from build123d import *

# Parameters (mm, degrees)
SKETCH063_W      = 2
SKETCH063_H      = 2
EXTRUDE068_DEPTH = 3.8
SKETCH062_W      = 2
SKETCH062_H      = 6.2
EXTRUDE067_DEPTH = 6.4
SKETCH061_W      = 2
SKETCH061_H      = 10.2
EXTRUDE066_DEPTH = 8.4


with BuildPart() as obj1:
    # Sketch063 → Extrude068 (new body, symmetric)
    with BuildSketch(Plane.XZ):
        with Locations((-2, 4.1)):
            Rectangle(SKETCH063_W, SKETCH063_H)
        with Locations((-2, -4.1)):
            Rectangle(SKETCH063_W, SKETCH063_H)
    extrude(amount=EXTRUDE068_DEPTH, both=True)


with BuildPart() as obj2:
    # Sketch062 → Extrude067 (new body, symmetric)
    with BuildSketch(Plane.XZ):
        Rectangle(SKETCH062_W, SKETCH062_H)
    extrude(amount=EXTRUDE067_DEPTH, both=True)


with BuildPart() as obj3:
    # Sketch061 → Extrude066 (new body, symmetric)
    with BuildSketch(Plane.XZ):
        Rectangle(SKETCH061_W, SKETCH061_H)
    extrude(amount=EXTRUDE066_DEPTH, both=True)

    # Cut036: cut obj2
    add(obj2.part, mode=Mode.SUBTRACT)

    # Fusion002: union obj1
    add(obj1.part)


solid = obj3.part
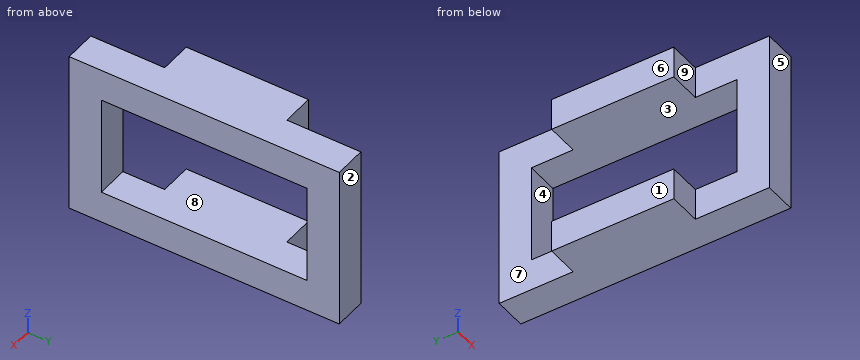
Read the model definition and answer for the solid it produces. Units are mm, in the model's axes. Face numbers are marked on the shaded views. A direction names the side the tool comes from. Round coordinates to 2 decimals unless told otherwise and drop trailing zeros. Loops run counter-clockwise (first coordinate to the right, second up) from the corner with the lowest first, then second, coordinate; pieces in that order, holes last.
Q1. Section B-B on x = 0.5 is taken. Write down the section's boundary in (y, z).
Q2. Each of these flat-tipped pins is pushed along its axis until it touches: pin 1 (2 mm diameter, centred on x = -1.5, z = -4, fed in from +Y); pin 2 (0.6 mm diameter, centred on x = -2.5, z = 4, fed in from +Y); pin 3 (1.4 mm diameter, centred on y = -6.5, z = 0, fed in from -X); pin 4 (2 mm diameter, centred on x = -2.5, z = -4.5, fed in from -Y). Where does it stop, or does it pass through?
Q3. Which of the six approach directions +Z, -Z, +X, -X, +Y, -Y give full straight-line access (tool end or side, diameter ignored) to the marked faces 5, 6, 7, 8 and 9?
Q4. Section D-D on z = -3.75 is taken. Write down the section's boundary in (x, y), and give its area (3 significant figures).
Q5. Section A-A on y = -5.5 is taken. Write down the section's boundary in (x, z).
Q6. Section C-C on z = -2.5 is taken. Write down the section's boundary in (x, y).
Q7. Consider probe 1 along Z at (x, y) = (-1.5, -2); probe 2 along Y at (x, z) = (-0.9, -2.75); probe 3 along X at (y, z) = (-6.75, 4). Determine where each line is inside the solid, lowest interval first.
Q8. Determine the mould class of the marked faces 1, 2, 3 and 4 for opening direction Y: released by +Y, released by -Y, zero draft, split by the parting line, or undercut.
Output:
1. outline: (-8.4, -5.1) - (8.4, -5.1) - (8.4, 5.1) - (-8.4, 5.1) - close; hole (-6.4, -3.1) - (6.4, -3.1) - (6.4, 3.1) - (-6.4, 3.1) - close
2. pin 1: stops at y = 8.4
2. pin 2: stops at y = 3.8
2. pin 3: stops at x = -1
2. pin 4: stops at y = -3.8
3. face 5: +Z, -Z, +X, -X, -Y
3. face 6: +Z, -Z, -X, +Y, -Y
3. face 7: +Z, -Z, -X, +Y
3. face 8: +X, -X
3. face 9: +Z, -Z, -X, -Y
4. outline: (-3, -3.8) - (-1, -3.8) - (-1, -8.4) - (1, -8.4) - (1, 8.4) - (-1, 8.4) - (-1, 3.8) - (-3, 3.8) - close
4. area: 48.8 mm2
5. outline: (-1, -5.1) - (1, -5.1) - (1, -3.1) - (-1, -3.1) - close; (-1, 3.1) - (1, 3.1) - (1, 5.1) - (-1, 5.1) - close
6. outline: (-1, -8.4) - (1, -8.4) - (1, -6.4) - (-1, -6.4) - close; (-1, 6.4) - (1, 6.4) - (1, 8.4) - (-1, 8.4) - close
7. probe 1: z = -5.1 to -3.1, 3.1 to 5.1
7. probe 2: y = -8.4 to -6.4, 6.4 to 8.4
7. probe 3: x = -1 to 1
8. face 1: zero draft
8. face 2: released by +Y
8. face 3: undercut
8. face 4: undercut
